from build123d import *

# Parameters (mm, degrees)
SKETCH1_R           = 25.4
BOSS_EXTRUDE1_DEPTH = 1.27
BOSS_EXTRUDE2_DEPTH = 1.27
SKETCH3_R           = 7.366
CUT_EXTRUDE1_DEPTH  = 10
CIRPATTERN1_COUNT   = 12
SKETCH4_R           = 18.283160809
CUT_EXTRUDE2_DEPTH  = 0.254


with BuildPart() as part:
    # Sketch1 → Boss-Extrude1 (new body)
    with BuildSketch(Plane.XY):
        Circle(SKETCH1_R)
    extrude(amount=BOSS_EXTRUDE1_DEPTH)

    # Sketch2 → Boss-Extrude2 (add)
    with BuildSketch(Plane.XY.offset(1.27)):
        with BuildLine():
            Line((-1.27, 31.75), (1.27, 31.75))
            Line((1.27, 31.75), (4.411023441, 25.014053494))
            ThreePointArc((4.411023441, 25.014053494), (0, 25.4), (-4.411023441, 25.014053494))
            Line((-4.411023441, 25.014053494), (-1.27, 31.75))
        make_face()
    boss_extrude2 = extrude(amount=-BOSS_EXTRUDE2_DEPTH)

    # Sketch3 → Cut-Extrude1 (cut)
    with BuildSketch(Plane(origin=(0, 0, 0), x_dir=(-1, 0, 0), z_dir=(0, 0, -1))):
        Circle(SKETCH3_R)
    extrude(amount=-CUT_EXTRUDE1_DEPTH, mode=Mode.SUBTRACT)

    # CirPattern1: Boss-Extrude2 ×12 about axis
    cirpattern1_axis = Axis((0, 0, 0), (0, 0, 1))
    for i in range(1, CIRPATTERN1_COUNT):
        add(boss_extrude2.rotate(cirpattern1_axis, i * 360 / CIRPATTERN1_COUNT))

    # Sketch4 → Cut-Extrude2 (cut)
    with BuildSketch(Plane(origin=(0, 0, 0), x_dir=(-1, 0, 0), z_dir=(0, 0, -1))):
        Circle(SKETCH4_R)
    extrude(amount=-CUT_EXTRUDE2_DEPTH, mode=Mode.SUBTRACT)


solid = part.part
The model under review builds one solid part; all positions refer to its coordinate system, in mm. A direction names the side the tool comes from. Coordinates: 2 decimals unless noted, no trailing zeros. Write each loop counter-clockwise with the first axis right and the second up, starting at its lowest first coordinate (ties: lowest second). Pieces come first, ordered by that corner, then holes. Notation, with made-up numbers: (16, 32) -> (24, 32) arc R20 ccw to (24, 70) -> close; hole circle Ø7 at (74.25, -22.75). An arc over 180 degrees is marked (long way). Answer in a Markdown table with one row per item.
1. Draft analysis for pull direction Y (two halves, no side actions). For faces 4 (the flat face through (-8, 0, 1.27)), 5 (the flat face through (26.03, 11.774, 0.644)), 6 (the flat face through (11.774, -26.03, 0.644)), 7 (the flat face through (2.82, 28.43, 0.64)), state which applies: +Y half, -Y half, draft (parallel to the pull), parting line (faces both ways), or undercut.
Answers below:
| item | result |
|---|---|
| face 4 | draft |
| face 5 | undercut |
| face 6 | -Y half |
| face 7 | +Y half |
2. We need section A-A, the plane y = 0. State the section outline as (x, z) points, and give its area (3 significant figures).
Answers below:
| item | result |
|---|---|
| outline | (-31.75, 0) -> (-18.28, 0) -> (-18.28, 0.25) -> (-7.37, 0.25) -> (-7.37, 1.27) -> (-31.75, 1.27) -> close; (7.37, 0.25) -> (18.28, 0.25) -> (18.28, 0) -> (31.75, 0) -> (31.75, 1.27) -> (7.37, 1.27) -> close |
| area | 56.4 mm^2 |
3. Wall thickness on probe 1 along Y at (x, z) = (0, 0.1); probe 2 along Y at (x, z) = (26.5, 1.15); probe 3 along Y at (x, z) = (27.5, 0.65): over which ranges is each line inside the solid? List them lowest first. Write a range as [from, to].
Answers below:
| item | result |
|---|---|
| probe 1 | y = [-31.75, -18.28], [18.28, 31.75] |
| probe 2 | y = [-16.94, -12.45], [-3.72, 3.72], [12.45, 16.94] |
| probe 3 | y = [-15.87, -13.87], [-3.25, 3.25], [13.87, 15.87] |
4. For faces 1 (the flat face through (-26.03, -11.774, 0.644)), 2 (the flat face through (-11.69, -25.97, 0.64)), 3 (the flat face through (11.69, 25.97, 0.64)), list the 3-axis set-ups (+Z, -Z, +X, -X, +Y, -Y) from which the entire face can be reached by the end or side of a thin tool; tool diameter is ignored.
Answers below:
| item | result |
|---|---|
| face 1 | +Z, -Z, -X |
| face 2 | +Z, -Z, -Y |
| face 3 | +Z, -Z, +Y |
5. Clearance check with a flat-ended pin moving along its axis: pin 1 Ø23.5 at (x, y) = (0, 0) entering from +Z. State where the tip first meets the part, or that it passes through.
Answers below:
| item | result |
|---|---|
| pin 1 | stops at z = 1.27 |
6. We need section C-C, the plane y = -15.5. State the section outline as (x, z) points, and give its area (3 significant figures).
Answers below:
| item | result |
|---|---|
| outline | (-27.71, 0) -> (-9.7, 0) -> (-9.7, 0.25) -> (9.7, 0.25) -> (9.7, 0) -> (27.71, 0) -> (27.71, 1.27) -> (-27.71, 1.27) -> close |
| area | 65.5 mm^2 |
